from build123d import *

# Parameters (mm, degrees)
SKETCH1_R           = 3.7592
BOSS_EXTRUDE1_DEPTH = 1.5875
CUT_EXTRUDE1_REACH  = 28.107
SKETCH2_W           = 3.302
SKETCH2_H           = 4.572
SKETCH2_H_2         = 3.7592


with BuildPart() as part:
    # Sketch1 → Boss-Extrude1 (new body)
    with BuildSketch(Plane.XY):
        with BuildLine():
            Line((11.112499999, 17.8308), (9.524999999, 17.8308))
            Line((9.524999999, 17.8308), (9.524999999, 19.05))
            Line((9.524999999, 19.05), (2.54, 19.05))
            ThreePointArc((2.54, 19.05), (-6.440256121, 15.330256121), (-10.16, 6.35))
            Line((-10.16, 6.35), (-10.16, 2.5908))
            Line((-10.160000001, 2.5908), (-11.747500001, 2.5908))
            Line((-11.747500001, 2.5908), (-11.747500001, 1.27))
            Line((-11.747500001, 1.27), (-10.160000001, 1.27))
            Line((-10.160000001, 1.27), (-10.160000001, -3.81))
            Line((-10.160000001, -3.81), (-17.78, -3.81))
            Line((-17.78, -3.81), (-17.78, -12.954))
            Line((-17.78, -12.954), (-10.16, -12.954))
            Line((-10.160000001, -12.954), (-10.160000001, -14.605))
            Line((-10.160000001, -14.605), (9.524999999, -14.605))
            Line((9.524999999, -14.605), (9.524999999, -6.4008))
            Line((9.524999999, -6.4008), (11.112499999, -6.4008))
            Line((11.112499999, -6.4008), (11.112499999, -5.08))
            Line((11.112499999, -5.08), (9.524999999, -5.08))
            Line((9.524999999, -5.08), (9.524999999, 2.54))
            Line((9.525, 2.54), (11.1125, 2.54))
            Line((11.1125, 2.54), (11.1125, 3.8608))
            Line((11.1125, 3.8608), (9.525, 3.8608))
            Line((9.524999999, 3.8608), (9.524999999, 16.51))
            Line((9.524999999, 16.51), (11.112499999, 16.51))
            Line((11.112499999, 16.51), (11.112499999, 17.8308))
        make_face()
        with BuildLine():
            ThreePointArc((-7.112, 6.35), (-4.284994652, 13.174994652), (2.54, 16.002))
            Line((2.54, 16.002), (5.968999999, 16.002))
            Line((5.968999999, 16.002), (5.968999999, 6.35))
            Line((5.968999999, 6.35), (-7.112, 6.35))
        make_face(mode=Mode.SUBTRACT)
        with BuildLine():
            ThreePointArc((-3.82905, -5.883688551), (4.572, -8.382), (-3.82905, -10.880311449))
            ThreePointArc((-3.82905, -10.880311449), (-7.874, -8.382), (-3.82905, -5.883688551))
        make_face(mode=Mode.SUBTRACT)
        Circle(SKETCH1_R, mode=Mode.SUBTRACT)
    extrude(amount=BOSS_EXTRUDE1_DEPTH)

    # Sketch2 → Cut-Extrude1 (cut, up to next)
    with BuildSketch(Plane.XY.offset(1.5875), mode=Mode.PRIVATE) as cut_extrude1_sk1:
        with Locations((7.873999999, -1.524)):
            Rectangle(SKETCH2_W, SKETCH2_H)
    cut_extrude1_tool1 = extrude(cut_extrude1_sk1.sketch, amount=-CUT_EXTRUDE1_REACH, mode=Mode.PRIVATE) & part.part
    # Sketch2 → Cut-Extrude1 (cut, up to next)
    with BuildSketch(Plane.XY.offset(1.5875), mode=Mode.PRIVATE) as cut_extrude1_sk2:
        with Locations((7.873999999, 19.7104)):
            Rectangle(SKETCH2_W, SKETCH2_H_2)
    cut_extrude1_tool2 = extrude(cut_extrude1_sk2.sketch, amount=-CUT_EXTRUDE1_REACH, mode=Mode.PRIVATE) & part.part
    add(cut_extrude1_tool1.solids().sort_by_distance((7.874, -1.524, 1.5875))[0], mode=Mode.SUBTRACT)
    add(cut_extrude1_tool2.solids().sort_by_distance((7.874, 19.7104, 1.5875))[0], mode=Mode.SUBTRACT)


solid = part.part
Work out the finished part from the listing and answer in its coordinate system (mm). A direction names the side the tool comes from. Round coordinates to 2 decimals unless told otherwise and drop trailing zeros. Write each loop counter-clockwise with the first axis right and the second up, starting at its lowest first coordinate (ties: lowest second). Pieces come first, ordered by that corner, then holes. Notation, with made-up numbers: (17, 13) -> (70, 13) arc R27 ccw to (70, 29) -> close; hole circle Ø6 at (74, 5). An arc over 180 degrees is marked (long way). Write each question's results on one line, items separated by ' | '.
Item 1: Flat-ended cylindrical pins translate along their axes: P1, Ø0.5, axis at x = 8, z = 1, coming from the +Y side; P2, Ø0.5, axis at x = -15.5, z = 1, coming from the -Y side; P3, Ø0.5, axis at y = 10, z = 1, coming from the -X side; P4, Ø5, axis at x = -11, y = 14.5, coming from the -Z side. Find the tip coordinate at first contact, or state that the pin passes through.
Result set:
P1: y = 17.83 | P2: y = -12.95 | P3: x = -9.7 | P4: through
Item 2: A cutting plane is placed at C-C, the plane x = -5.08. Count the separate pieces of the cut face and the enclosed holes in it, plus the area to 3 significant figures.
Result set:
separate pieces: 3 | enclosed holes: 0 | area: 31.1 mm^2
Item 3: A cutting plane is placed at A-A, the plane x = 7.5. Determine the outline of the cut face in (y, z) (1 decimal).
Result set:
outline: (-14.6, 0) -> (-3.8, 0) -> (-3.8, 1.6) -> (-14.6, 1.6) -> close; (0.8, 0) -> (17.8, 0) -> (17.8, 1.6) -> (0.8, 1.6) -> close
Item 4: Which of the six approach directions +Z, -Z, +X, -X, +Y, -Y give full straight-line access (tool end or side, diameter ignored) to faces 5 (the face through (-10.16, -1, 1)), 6 (the face through (9.525, -11, 1)), 7 (the face through (-11, 2.591, 1))?
Result set:
face 5: +Z, -Z, -X | face 6: +Z, -Z, +X, -Y | face 7: +Z, -Z, -X, +Y
Item 5: A cutting plane is placed at B-B, the plane y = 0. Determine the outline of the cut face in (x, z).
Result set:
outline: (-10.16, 0) -> (-3.76, 0) -> (-3.76, 1.59) -> (-10.16, 1.59) -> close; (3.76, 0) -> (6.22, 0) -> (6.22, 1.59) -> (3.76, 1.59) -> close
Item 6: The mould has two halves that part along Y. Classify faces 1 (the face through (9.525, 2, 1)), 2 (the face through (-14, -12.954, 1)), 3 (the face through (-10.16, 4, 1)), 4 (the face through (10, 16.51, 1)): +Y half, -Y half, draft (parallel to the pull), parting line (faces both ways), or undercut.
Result set:
face 1: undercut | face 2: -Y half | face 3: draft | face 4: undercut
Item 7: Find the intervals of material crossed by line 1 along Y through (x, z) = (-11.5, 0.35); line 2 along Y through (x, z) = (1, 1.3) (3 decimals); line 3 along Y through (x, z) = (-5.08, 1.2) (3 decimals), in increasing order. Write a range as [from, to].
Result set:
line 1: [-12.95, -3.81], [1.27, 2.59] | line 2: [-14.605, -12.843], [-3.921, -3.624], [3.624, 6.35], [15.878, 18.956] | line 3: [-14.605, -11.176], [-5.588, 6.35], [12.274, 16.51]
